Here's the drawing with two shaded views (mm, measured from the low corner). I have some questions. Round coordinates to 2 decimals unless told otherwise and drop trailing zeros. Loops run counter-clockwise (first coordinate to the right, second up) from the corner with the lowest first, then second, coordinate; pieces in that order, holes last. Notation, with made-up numbers: M 54,37 L 98,37 A6 cw 98,45 Z; hole C 34.5,30.5 d7. An arc over 180 degrees is marked long. Answer as CSV lines item,"result".
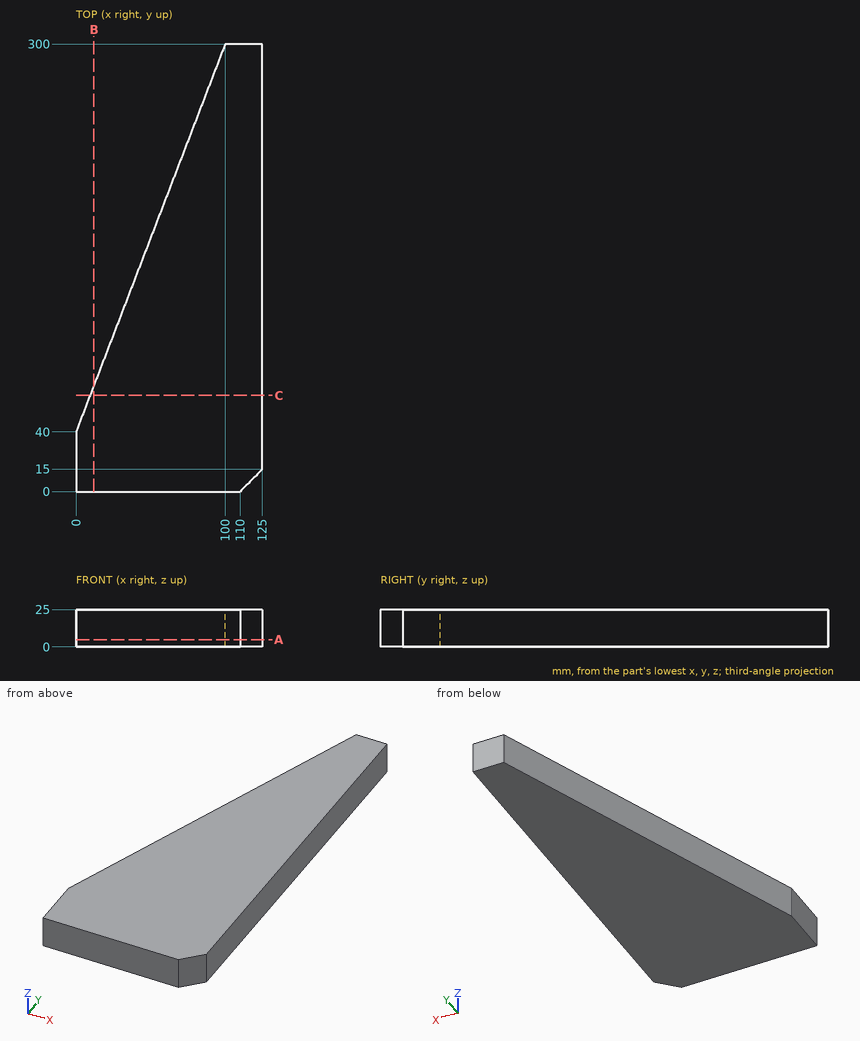
1. I want a section at A-A, the plane z = 4.75. Please give me the cut outline in (x, y), and give its area (3 significant figures).
Evaluation:
outline,"M 0,0 L 110,0 L 125,15 L 125,300 L 100,300 L 0,40 Z"
area,"24,400 mm²"
2. I want a section at B-B, the plane x = 12. Please give me the cut outline in (y, z).
Evaluation:
outline,"M 0,0 L 71.2,0 L 71.2,25 L 0,25 Z"
3. If I drill on line 1 (X direction, y = 207, z = 17.75); line 2 (X direction, y = 73.5, z = 23.5); line 3 (Y direction, x = 115, z = 7.5), over which ranges is the centre line in solid material (lowest first)? Write a range as [from, to].
Evaluation:
line 1,"x = [64.23, 125]"
line 2,"x = [12.88, 125]"
line 3,"y = [5, 300]"
4. I want a section at C-C, the plane y = 64.5. Please give me the cut outline in (x, z), and give its area (3 significant figures).
Evaluation:
outline,"M 9.42,0 L 125,0 L 125,25 L 9.42,25 Z"
area,"2,890 mm²"
